from build123d import *

# Parameters (mm, degrees)
SKETCH2_W                      = 31.75
SKETCH2_H                      = 50.8
BASE_FLANGE1_DEPTH             = 2.54
EDGE_FLANGE1_STRIP_W           = 11.6332
EDGE_FLANGE1_STRIP_H           = 2.54
EDGE_FLANGE1_STRIP_CUT_DEPTH   = 50.8
EDGE_FLANGE1_STRIP_2_W         = 11.6332
EDGE_FLANGE1_STRIP_2_H         = 2.54
EDGE_FLANGE1_STRIP_CUT_2_DEPTH = 50.8
EDGE_FLANGE1_DEPTH             = 50.8
EDGE_FLANGE1_BEND_DEPTH        = 50.8
CUT_EXTRUDE1_DEPTH             = 58.487669113
BOSS_EXTRUDE1_START            = -2.54
SKETCH14_R                     = 6.35
BOSS_EXTRUDE1_DEPTH            = 27.94
SKETCH15_R                     = 6.35
BOSS_EXTRUDE2_DEPTH            = 2.54
SKETCH16_R                     = 8.255
BOSS_EXTRUDE3_DEPTH            = 2.54


# Sheet-metal steps are written as plain solids
with BuildPart() as part:
    # Sketch2 → Base-Flange1 (new body)
    with BuildSketch(Plane(origin=(0, 0, 0), x_dir=(1, 0, 0), z_dir=(0, 1, 0))):
        Rectangle(SKETCH2_W, SKETCH2_H)
    extrude(amount=-BASE_FLANGE1_DEPTH)

    # Edge-Flange1 strip (across the edge) → Edge-Flange1 strip cut (cut)
    with BuildSketch(Plane(origin=(15.875, -2.54, -25.4), x_dir=(-1, 0, 0), z_dir=(0, 0, 1))):
        with Locations((-2.54, -1.27)):
            Rectangle(EDGE_FLANGE1_STRIP_W, EDGE_FLANGE1_STRIP_H)
    extrude(amount=EDGE_FLANGE1_STRIP_CUT_DEPTH, mode=Mode.SUBTRACT)

    # Edge-Flange1 strip 2 (across the edge) → Edge-Flange1 strip cut 2 (cut)
    with BuildSketch(Plane(origin=(-15.875, -2.54, 25.4), x_dir=(1, 0, 0), z_dir=(0, 0, -1))):
        with Locations((-2.54, -1.27)):
            Rectangle(EDGE_FLANGE1_STRIP_2_W, EDGE_FLANGE1_STRIP_2_H)
    extrude(amount=EDGE_FLANGE1_STRIP_CUT_2_DEPTH, mode=Mode.SUBTRACT)

    # Edge-Flange1 section (across the edge) → Edge-Flange1 (add)
    with BuildSketch(Plane(origin=(15.875, -2.54, -25.4), x_dir=(-1, 0, 0), z_dir=(0, 0, 1))):
        with BuildLine():
            Line((0, 0.7366), (0, 38.1))
            Line((0, 38.1), (2.54, 38.1))
            Line((2.54, 38.1), (2.54, 0.7366))
            ThreePointArc((2.54, 0.7366), (2.755745145, 0.215745145), (3.2766, 0))
            Line((3.2766, 0), (3.2766, -2.54))
            ThreePointArc((3.2766, -2.54), (0.959693921, -1.580306079), (0, 0.7366))
        make_face()
    extrude(amount=EDGE_FLANGE1_DEPTH)

    # Edge-Flange1 section 2 (across the edge) → Edge-Flange1 bend (add)
    with BuildSketch(Plane(origin=(-15.875, -2.54, 25.4), x_dir=(1, 0, 0), z_dir=(0, 0, -1))):
        with BuildLine():
            Line((0, 0.7366), (0, 38.1))
            Line((0, 38.1), (2.54, 38.1))
            Line((2.54, 38.1), (2.54, 0.7366))
            ThreePointArc((2.54, 0.7366), (2.755745145, 0.215745145), (3.2766, 0))
            Line((3.2766, 0), (3.2766, -2.54))
            ThreePointArc((3.2766, -2.54), (0.959693921, -1.580306079), (0, 0.7366))
        make_face()
    extrude(amount=EDGE_FLANGE1_BEND_DEPTH)

    # Sketch13 → Cut-Extrude1 (cut, through all)
    with BuildSketch(Plane(origin=(15.875, 0, 0), x_dir=(0, 0, -1), z_dir=(1, 0, 0))):
        with BuildLine():
            Line((-25.4, -40.64), (3e-08, -40.64))
            ThreePointArc((3e-08, -40.64), (-6.840376035, -38.640432501), (-11.526768838, -33.271378824))
            Line((-11.526768838, -33.271378824), (-25.4, -3.2766))
            Line((-25.4, -3.2766), (-25.4, -40.64))
        make_face()
        with BuildLine():
            Line((25.4, -3.2766), (11.526768838, -33.271378824))
            ThreePointArc((11.526768838, -33.271378824), (6.84037606, -38.640432485), (3e-08, -40.64))
            Line((3e-08, -40.64), (25.4, -40.64))
            Line((25.4, -40.64), (25.4, -3.2766))
        make_face()
    extrude(amount=-CUT_EXTRUDE1_DEPTH, mode=Mode.SUBTRACT)

    # Sketch14 → Boss-Extrude1 (add)
    with BuildSketch(Plane(origin=(15.875, 0, 0), x_dir=(0, 0, -1), z_dir=(1, 0, 0)).offset(BOSS_EXTRUDE1_START)):
        with Locations(Location((0, -27.94, 0), (0, 0, 90))):
            Circle(SKETCH14_R)
    extrude(amount=-BOSS_EXTRUDE1_DEPTH)

    # Sketch15 → Boss-Extrude2 (add)
    with BuildSketch(Plane(origin=(0, 0, 0), x_dir=(1, 0, 0), z_dir=(0, 1, 0))):
        with Locations(Location((0, 0, 0), (0, 0, 270))):
            Circle(SKETCH15_R)
    extrude(amount=BOSS_EXTRUDE2_DEPTH)

    # Sketch16 → Boss-Extrude3 (add)
    with BuildSketch(Plane(origin=(0, 2.54, 0), x_dir=(1, 0, 0), z_dir=(0, 1, 0))):
        with Locations(Location((0, 0, 0), (0, 0, 270))):
            Circle(SKETCH16_R)
    extrude(amount=BOSS_EXTRUDE3_DEPTH)


solid = part.part
Geometry check sheet. Reference: the model listing, model coordinates, mm. A direction names the side the tool comes from. Coordinates: 2 decimals unless noted, no trailing zeros. Order: outer loops, then holes, each group sorted by start corner. A loop starts at its lowest first (then second) coordinate and runs counter-clockwise, first axis right, second up. Notation, with made-up numbers: (13, 35) -> (34, 35) arc R20 cw to (34, 40) -> close; hole circle Ø11 at (80.25, 56.5). An arc over 180 degrees is marked (long way). Use a Markdown table: item, result. Add a question column.
1. Mould release check, pull along Y, two halves, no side actions. Record for faces 4 (the face through (-5.023, 3.792, -6.551)), 5 (the face through (14.623, -18.064, -18.56)), 6 (the face through (-3.86, 1.25, -5.04)), 7 (the face through (13.335, -18, 0)): pulls with the +Y half, pulls with the -Y half, needs draft (parallel to the pull), parting line crosses it, or undercut.
2. Go/stop test with flat-tipped pins: pin 1 Ø18 at (x, z) = (2.5, 0.5) entering from -Y; pin 2 Ø3 at (x, y) = (-4, -20) entering from -Z; pin 3 Ø8 at (x, z) = (-7.5, -12) entering from -Y; pin 4 Ø7.5 at (x, z) = (-6, -4.5) entering from -Y. Record where each tip stops, or that it passes through.
3. Cross-section at D-D (y = -27). Enter the section's corners in (x, z) (3 decimals), and give its area (3 significant figures).
4. Cross-section at B-B (y = -9). Enter the section's corners in (x, z) (3 decimals).
5. Cross-section at A-A (x = 0). Enter the section's corners in (y, z) (3 decimals), and give its area (3 significant figures).
6. Cross-section at C-C (z = 13). Enter the section's corners in (x, y) (3 decimals).
7. Set-up check for faces 1 (the face through (0, -2.54, 0)), 2 (the face through (-14.89, -0.934, 0.356)), 3 (the face through (-6.1, 2.54, 2.4)): record each of +Z, -Z, +X, -X, +Y, -Y from which the full face is reachable in a straight line by a thin tool's end or side.
8. Material ranges on L1, parallel to X at y = -21.5, z = -4 (3 decimals); L2, parallel to Y at x = -1, z = -8; L3, parallel to Y at x = -4, z = -20, recorded low to high.
Filled sheet:
| question | item | result |
|---|---|---|
| 1 | face 4 | needs draft |
| 1 | face 5 | pulls with the -Y half |
| 1 | face 6 | undercut |
| 1 | face 7 | undercut |
| 2 | pin 1 | y = -34.29 |
| 2 | pin 2 | through |
| 2 | pin 3 | y = -2.54 |
| 2 | pin 4 | y = -34.25 |
| 3 | outline | (-15.875, -14.427) -> (-13.335, -14.427) -> (-13.335, -6.28) -> (13.335, -6.28) -> (13.335, -14.427) -> (15.875, -14.427) -> (15.875, 14.427) -> (13.335, 14.427) -> (13.335, 6.28) -> (-13.335, 6.28) -> (-13.335, 14.427) -> (-15.875, 14.427) -> close |
| 3 | area | 482 mm2 |
| 4 | outline | (-15.875, -22.753) -> (-13.335, -22.753) -> (-13.335, 22.753) -> (-15.875, 22.753) -> close; (13.335, -22.753) -> (15.875, -22.753) -> (15.875, 22.753) -> (13.335, 22.753) -> close |
| 5 | outline | circle Ø12.7 at (-27.94, 0); (-2.54, -25.4) -> (0, -25.4) -> (0, -6.35) -> (2.54, -6.35) -> (2.54, -8.255) -> (5.08, -8.255) -> (5.08, 8.255) -> (2.54, 8.255) -> (2.54, 6.35) -> (0, 6.35) -> (0, 25.4) -> (-2.54, 25.4) -> close |
| 5 | area | 330 mm2 |
| 6 | outline | (-15.875, -30.086) -> (-13.335, -30.086) -> (-13.335, -3.277) arc R0.737 cw to (-12.598, -2.54) -> (12.598, -2.54) arc R0.737 cw to (13.335, -3.277) -> (13.335, -30.086) -> (15.875, -30.086) -> (15.875, -3.277) arc R3.277 ccw to (12.598, 0) -> (-12.598, 0) arc R3.277 ccw to (-15.875, -3.277) -> close |
| 7 | face 1 | +Z, -Z |
| 7 | face 2 | +Z, -Z, -X, +Y |
| 7 | face 3 | none |
| 8 | L1 | -15.875 to -13.335, 13.335 to 15.875 |
| 8 | L2 | -2.54 to 0, 2.54 to 5.08 |
| 8 | L3 | -2.54 to 0 |
